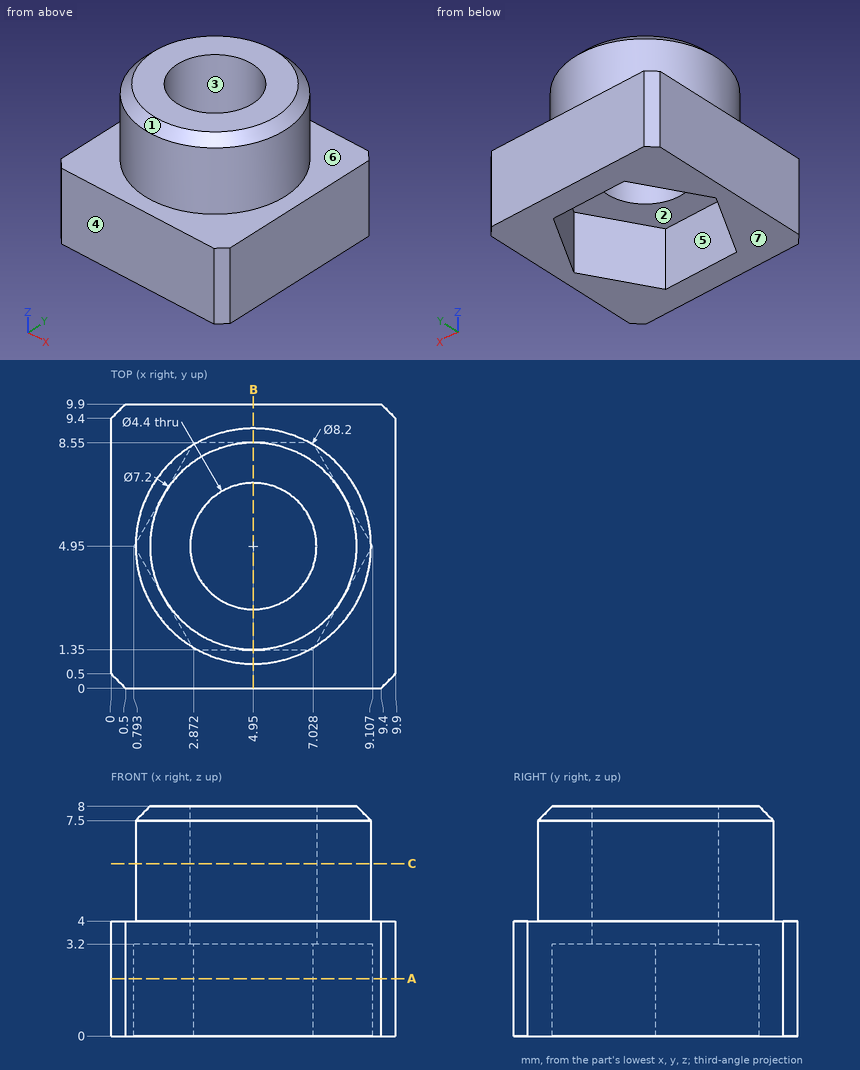
Here's the drawing with two shaded views (mm, measured from the low corner). I have some questions. A direction names the side the tool comes from. Coordinates: 2 decimals unless noted, no trailing zeros. Write each loop counter-clockwise with the first axis right and the second up, starting at its lowest first coordinate (ties: lowest second). Pieces come first, ordered by that corner, then holes. Notation, with made-up numbers: (-29.5, 69) -> (13.5, 69) arc R11 ccw to (13.5, 81) -> close; hole circle Ø2 at (17, 55). An arc over 180 degrees is marked (long way). One line per question, with ' | ' between items. Start each with the question number.
1. Please list where these lines run through material, in increasing order: line 1 along Y through (x, z) = (4.95, 4.9); line 2 along Y through (x, z) = (4.5, 2); line 3 along Z through (x, y) = (1.75, 8).
2. If we section it at A-A (z = 2): Please give me the cut outline in (x, y).
3. For the marked faces 5, 6 and 7, which set-ups out of +Z, -Z, +X, -X, +Y, -Y let a thin tool reach every point of the face, with its end or its side?
4. If we section it at B-B (x = 4.95): Please give me the cut outline in (y, z).
5. If we section it at C-C (z = 6): Please give me the cut outline in (x, y), and give its area (3 significant figures).
6. Will these pins go through, and if not, where does the flat tip stop? P1, Ø5, axis at x = 4.95, y = 4.95, coming from the -Z side; P2, Ø2, axis at x = 8, z = 6, coming from the +Y side; P3, Ø1.5, axis at y = 6, z = 6, coming from the -X side.
7. Thinking about a two-plate mould opening in Y: for the marked faces 1, 2, 3 and 4, which applies, pulls with the +Y half, pulls with the -Y half, needs draft (parallel to the pull), parting line crosses it, or undercut?
Return value:
1) line 1: y = 0.85 to 2.75, 7.15 to 9.05 | line 2: y = 0 to 1.35, 8.55 to 9.9 | line 3: z = 0 to 4
2) outline: (0, 0.5) -> (0.5, 0) -> (9.4, 0) -> (9.9, 0.5) -> (9.9, 9.4) -> (9.4, 9.9) -> (0.5, 9.9) -> (0, 9.4) -> close; hole (0.79, 4.95) -> (2.87, 1.35) -> (7.03, 1.35) -> (9.11, 4.95) -> (7.03, 8.55) -> (2.87, 8.55) -> close
3) face 5: -Z | face 6: +Z | face 7: -Z, +X, -X, +Y, -Y
4) outline: (0, 0) -> (1.35, 0) -> (1.35, 3.2) -> (2.75, 3.2) -> (2.75, 8) -> (1.35, 8) -> (0.85, 7.5) -> (0.85, 4) -> (0, 4) -> close; (7.15, 3.2) -> (8.55, 3.2) -> (8.55, 0) -> (9.9, 0) -> (9.9, 4) -> (9.05, 4) -> (9.05, 7.5) -> (8.55, 8) -> (7.15, 8) -> close
5) outline: circle Ø8.2 at (4.95, 4.95); hole circle Ø4.4 at (4.95, 4.95) | area: 37.6 mm²
6) P1: stops at z = 3.2 | P2: stops at y = 8.5 | P3: stops at x = 0.86
7) face 1: parting line crosses it | face 2: undercut | face 3: undercut | face 4: pulls with the -Y half
